Design review of the part built by this model. Coordinates are the model's own, in mm. A direction names the side the tool comes from. Give positions to 0.01 mm unless a question says otherwise; leave off trailing zeros. Order: outer loops, then holes, each group sorted by start corner. A loop starts at its lowest first (then second) coordinate and runs counter-clockwise, first axis right, second up. Notation, with made-up numbers: (74, -10) -> (96, -10) arc R31 ccw to (96, 14) -> close; hole circle Ø3 at (79.25, -38). An arc over 180 degrees is marked (long way). Return JSON: item names as keys, results as strings.
```python
from build123d import *

# Parameters (mm, degrees)
SKETCH1_W           = 150
SKETCH1_H           = 150
BOSS_EXTRUDE1_DEPTH = 10
SKETCH3_W           = 100
SKETCH3_H           = 50
BOSS_EXTRUDE2_DEPTH = 50
CUT_EXTRUDE1_DEPTH  = 205.266982158
SKETCH5_W           = 100
SKETCH5_H           = 50
CUT_EXTRUDE2_DEPTH  = 218.944947177
SKETCH7_W           = 120
SKETCH7_H           = 70
BOSS_EXTRUDE6_DEPTH = 50
BOSS_EXTRUDE7_DEPTH = 100
SKETCH9_W           = 100
SKETCH9_H           = 40
CUT_EXTRUDE4_DEPTH  = 40
BOSS_EXTRUDE8_DEPTH = 100
CUT_EXTRUDE5_DEPTH  = 211.535032714
SHELL1_START        = 35
SHELL1_DEPTH        = 80


# Read off the part's stored shape, not the designer's step: Shell1
with BuildPart() as part:
    # Sketch1 → Boss-Extrude1 (new body)
    with BuildSketch(Plane(origin=(0, 0, 0), x_dir=(1, 0, 0), z_dir=(0, 1, 0))):
        with Locations((75, 75)):
            Rectangle(SKETCH1_W, SKETCH1_H)
    extrude(amount=BOSS_EXTRUDE1_DEPTH)

    # Sketch3 → Boss-Extrude2 (add)
    with BuildSketch(Plane(origin=(0, 10, 0), x_dir=(1, 0, 0), z_dir=(0, 1, 0))):
        with Locations((75, 100)):
            Rectangle(SKETCH3_W, SKETCH3_H)
    extrude(amount=BOSS_EXTRUDE2_DEPTH)

    # Sketch4 → Cut-Extrude1 (cut, through all)
    with BuildSketch(Plane.ZY.offset(-25)):
        Polygon((-125, 60), (-75, 10), (-75, 60), align=None)
    extrude(amount=-CUT_EXTRUDE1_DEPTH, mode=Mode.SUBTRACT)

    # Sketch5 → Cut-Extrude2 (cut, through all)
    with BuildSketch(Plane(origin=(0, 10, 0), x_dir=(1, 0, 0), z_dir=(0, 1, 0))):
        with Locations((75, 50)):
            Rectangle(SKETCH5_W, SKETCH5_H)
    extrude(amount=-CUT_EXTRUDE2_DEPTH, mode=Mode.SUBTRACT)

    # Sketch7 → Boss-Extrude6 (add)
    with BuildSketch(Plane.XZ):
        with Locations((75, -50)):
            Rectangle(SKETCH7_W, SKETCH7_H)
    extrude(amount=BOSS_EXTRUDE6_DEPTH)

    # Sketch6 → Boss-Extrude7 (add)
    with BuildSketch(Plane(origin=(25, 0, 0), x_dir=(0, 0, -1), z_dir=(1, 0, 0))):
        Polygon((75, 0), (75, 10), (65, 0), align=None)
    extrude(amount=BOSS_EXTRUDE7_DEPTH)

    # Sketch9 → Cut-Extrude4 (cut)
    with BuildSketch(Plane(origin=(0, 0, 0), x_dir=(1, 0, 0), z_dir=(0, 1, 0))):
        with Locations((75, 45)):
            Rectangle(SKETCH9_W, SKETCH9_H)
    extrude(amount=-CUT_EXTRUDE4_DEPTH, mode=Mode.SUBTRACT)

    # Sketch10 → Boss-Extrude8 (add)
    with BuildSketch(Plane(origin=(25, 0, 0), x_dir=(0, 0, -1), z_dir=(1, 0, 0))):
        Polygon((65, 0), (25, -40), (65, -40), align=None)
    extrude(amount=BOSS_EXTRUDE8_DEPTH)

    # Sketch11 → Cut-Extrude5 (cut, through all)
    with BuildSketch(Plane(origin=(135, 0, 0), x_dir=(0, 0, -1), z_dir=(1, 0, 0))):
        Polygon((85, 0), (85, -50), (35, -50), align=None)
    extrude(amount=-CUT_EXTRUDE5_DEPTH, mode=Mode.SUBTRACT)

    # Shell1 outline → Shell1 (cut)
    with BuildSketch(Plane.YZ.offset(SHELL1_START)):
        Polygon((45.857864376, -125), (10, -89.142135624), (10, -125), align=None)
    extrude(amount=SHELL1_DEPTH, mode=Mode.SUBTRACT)


solid = part.part
```
Item 1: Mouldability with a two-part tool opening along Y and no side actions: class faces 5 (the face through (115, 20, -115)), 6 (the face through (135, -19, -43)), 7 (the face through (74, 11, -76)) as released by +Y, released by -Y, zero draft, split by the parting line, or undercut.
Result set:
{"face 5": "undercut", "face 6": "zero draft", "face 7": "released by +Y"}
Item 2: For pin 1 (4 mm diameter, centred on x = 112.5, z = -121, fed in from +Y); pin 2 (12 mm diameter, centred on x = 124.5, z = -28.5, fed in from +Y); pin 3 (5 mm diameter, centred on x = 116, y = 20.5, fed in from +Z), all flat-tipped, find the tip position at first contact; note any pin that passes through.
Result set:
{"pin 1": "stops at y = 58", "pin 2": "stops at y = 10", "pin 3": "stops at z = -83"}
Item 3: Add section C-C (z = -113). Give the boundary of the cut face in (x, y), plus the area to 3 significant figures.
Result set:
{"outline": "(0, 0) -> (150, 0) -> (150, 10) -> (125, 10) -> (125, 48) -> (25, 48) -> (25, 10) -> (0, 10) -> close; hole (35, 10) -> (115, 10) -> (115, 33.86) -> (35, 33.86) -> close", "area": "3,390 mm^2"}
Item 4: Machinability: for faces 1 (the face through (35, 20, -115)), 2 (the face through (125, -9, -44)), 3 (the face through (125, 24, -111)), 4 (the face through (74, 51, -125)), which of the approach directions +Z, -Z, +X, -X, +Y, -Y give a long, thin tool a straight path to every point of the face, cutting with its end or side? Answer none if there is none.
Result set:
{"face 1": "-Z", "face 2": "+Y", "face 3": "+Z, -Z, +X, +Y", "face 4": "-Z, +X, -X, +Y"}
Item 5: Add section A-A (z = -60.5). Give the boundary of the cut face in (x, y), plus the area to 3 significant figures.
Result set:
{"outline": "(0, 0) -> (15, 0) -> (15, -24.5) -> (135, -24.5) -> (135, 0) -> (150, 0) -> (150, 10) -> (125, 10) -> (125, -4.5) -> (25, -4.5) -> (25, 10) -> (0, 10) -> close", "area": "2,990 mm^2"}
Item 6: Wall thickness on L1, parallel to X at y = -25, z = -32.5; L2, parallel to X at y = 8.5, z = -54; L3, parallel to Y at x = 53, z = -137: over which ranges is each line inside the solid? List them lowest first. Write a range as [from, to].
Result set:
{"L1": "x = [15, 25], [125, 135]", "L2": "x = [0, 25], [125, 150]", "L3": "y = [0, 10]"}
Item 7: Add section D-D (x = 60.5). Give the boundary of the cut face in (y, z), plus the area to 3 significant figures.
Result set:
{"outline": "(-50, -35) -> (0, -85) -> (0, -150) -> (10, -150) -> (10, -89.14) -> (45.86, -125) -> (60, -125) -> (-40, -25) -> (10, -25) -> (10, 0) -> (0, 0) -> (0, -15) -> (-50, -15) -> close", "area": "3,110 mm^2"}
Item 8: Add section B-B (y = 4). Give the boundary of the cut face in (x, z).
Result set:
{"outline": "(0, -150) -> (150, -150) -> (150, 0) -> (0, 0) -> close; hole (25, -69) -> (125, -69) -> (125, -25) -> (25, -25) -> close"}
